```python
from build123d import *

# Parameters (mm, degrees)
F1_DEPTH = 76.2
F2_W     = 66.04
F2_H     = 38.1
F3_DEPTH = 787.4
F4_R     = 12.7
F5_DEPTH = 78.74


with BuildPart() as f1:
    # F0 (on Front) → F1 (new body)
    with BuildSketch(Plane.XZ):
        Polygon((116.84, 152.4), (0, 152.4), (0, 0), (254, 0), (254, 63.5), (116.84, 63.5), align=None)
    extrude(amount=F1_DEPTH)

    # F2 (on face) → F3 (cut)
    with BuildSketch(Plane.XZ.offset(76.2)):
        with Locations((58.42, 107.95)):
            Rectangle(F2_W, F2_H)
    extrude(amount=-F3_DEPTH, mode=Mode.SUBTRACT)

    # F4 (on face) → F5 (cut)
    with BuildSketch(Plane.XZ.offset(76.2)):
        with Locations((50.8, 33.02)):
            Circle(F4_R)
        with Locations((203.2, 33.02)):
            Circle(F4_R)
    extrude(amount=-F5_DEPTH, mode=Mode.SUBTRACT)


solid = f1.part
```
Geometry check sheet. Reference: the model listing, model coordinates, mm. A direction names the side the tool comes from. Give positions to 0.01 mm unless a question says otherwise; leave off trailing zeros. Write each loop counter-clockwise with the first axis right and the second up, starting at its lowest first coordinate (ties: lowest second). Pieces come first, ordered by that corner, then holes. Notation, with made-up numbers: (59, -13.75) - (93, -13.75) arc R23 cw to (93, 8.25) - close; hole circle Ø7 at (-10, 45). An arc over 180 degrees is marked (long way). Use a Markdown table: item, result.
Q1. Section check B-B, the plane x = 50.8. Enter the section's corners in (y, z).
Computed:
| item | result |
|---|---|
| outline | (-76.2, 0) - (0, 0) - (0, 20.32) - (-76.2, 20.32) - close; (-76.2, 45.72) - (0, 45.72) - (0, 88.9) - (-76.2, 88.9) - close; (-76.2, 127) - (0, 127) - (0, 152.4) - (-76.2, 152.4) - close |
Q2. Draft check along X on faces 1 (the face through (58, -39, 127)), 2 (the face through (41.44, -38.633, 41.603)), 3 (the face through (254, -38, 31)), 4 (the face through (125, -38, 0)). Enter one of: pulls with the +X half, pulls with the -X half, needs draft (parallel to the pull), parting line crosses it, or undercut.
Computed:
| item | result |
|---|---|
| face 1 | undercut |
| face 2 | undercut |
| face 3 | pulls with the +X half |
| face 4 | needs draft |
Q3. Set-up check for faces 5 (the face through (97, 0, 60)), 6 (the face through (58, -39, 88.9)), 7 (the face through (186, -38, 63.5)): record each of +Z, -Z, +X, -X, +Y, -Y from which the full face is reachable in a straight line by a thin tool's end or side.
Computed:
| item | result |
|---|---|
| face 5 | +Z, -Z, +X, -X, +Y |
| face 6 | +Y, -Y |
| face 7 | +Z, +X, +Y, -Y |
Q4. Go/stop test with flat-tipped pins: P1, Ø11.5, axis at y = -35, z = 98.5, coming from the -X side; P2, Ø23, axis at x = 209, y = -54, coming from the +Z side; P3, Ø4, axis at y = -9, z = 76, coming from the +X side. Record where each tip stops, or that it passes through.
Computed:
| item | result |
|---|---|
| P1 | stops at x = 0 |
| P2 | stops at z = 63.5 |
| P3 | stops at x = 116.84 |
Q5. Section check C-C, the plane y = -6. Enter the section's corners in (x, z).
Computed:
| item | result |
|---|---|
| outline | (0, 0) - (254, 0) - (254, 63.5) - (116.84, 63.5) - (116.84, 152.4) - (0, 152.4) - close; hole (25.4, 88.9) - (91.44, 88.9) - (91.44, 127) - (25.4, 127) - close; hole circle Ø25.4 at (50.8, 33.02); hole circle Ø25.4 at (203.2, 33.02) |
Q6. Section check D-D, the plane z = 33.02. Enter the section's corners in (x, y), then the cut area to 3 significant figures.
Computed:
| item | result |
|---|---|
| outline | (0, -76.2) - (38.1, -76.2) - (38.1, 0) - (0, 0) - close; (63.5, -76.2) - (190.5, -76.2) - (190.5, 0) - (63.5, 0) - close; (215.9, -76.2) - (254, -76.2) - (254, 0) - (215.9, 0) - close |
| area | 15,500 mm² |
Q7. Section check A-A, the plane z = 100. Enter the section's corners in (x, y), then the cut area to 3 significant figures.
Computed:
| item | result |
|---|---|
| outline | (0, -76.2) - (25.4, -76.2) - (25.4, 0) - (0, 0) - close; (91.44, -76.2) - (116.84, -76.2) - (116.84, 0) - (91.44, 0) - close |
| area | 3,870 mm² |
Q8. Thickness scan on L1, parallel to Z at x = 50.8, y = -45.5; L2, parallel to Z at x = 203, y = -27; L3, parallel to Z at x = 29.5, y = -23. Record the ranges inside material, lowest first. Write a range as [from, to].
Computed:
| item | result |
|---|---|
| L1 | z = [0, 20.32], [45.72, 88.9], [127, 152.4] |
| L2 | z = [0, 20.32], [45.72, 63.5] |
| L3 | z = [0, 88.9], [127, 152.4] |
